CAD build for the part. Positions are in the model's coordinates, mm. Face numbers are marked on the shaded views. A direction names the side the tool comes from. Round coordinates to 2 decimals unless told otherwise and drop trailing zeros. Write each loop counter-clockwise with the first axis right and the second up, starting at its lowest first coordinate (ties: lowest second). Pieces come first, ordered by that corner, then holes. Notation, with made-up numbers: (-20.75, 75.25) - (22.25, 75.25) arc R20 ccw to (22.25, 109.25) - close; hole circle Ø1 at (30.5, 76). An arc over 180 degrees is marked (long way). Use one line per item in the form item = value. Start each with the question number.
Item 1: Pin check, flat tips, straight feed: pin 1 (1.8 mm diameter, centred on x = -13.5, z = 4, fed in from +Y); pin 2 (1.2 mm diameter, centred on x = -0.5, y = 1, fed in from -Z); pin 3 (0.8 mm diameter, centred on x = 1, y = 0.5, fed in from +Z). Stop position of each tip, or through.
Item 2: Band-saw the part on B-B, the plane z = 4. List the corners of the cut face in (x, y).
Item 3: Band-saw the part on D-D, the plane x = 6.5. List the corners of the cut face in (y, z).
Item 4: Band-saw the part on C-C, the plane x = 14.5. List the corners of the cut face in (y, z), and give its area (3 significant figures).
Item 5: Tool access for the marked faces 5, 6 and 7: list every direction of +Z, -Z, +X, -X, +Y, -Y with a clear straight run to the whole face (end or side of a thin tool).
Item 6: Band-saw the part on A-A, the plane x = -11.5. List the corners of the cut face in (y, z), and give its area (3 significant figures).
Item 7: Drill centre lines: L1, parallel to X at y = 7.5, z = 4.5; L2, parallel to Y at x = -4.3, z = 3; L3, parallel to Y at x = 6, z = 1.25. Where is each one in solid material? Low to high.
Item 8: Pull direction X, two halves, no side cores. Call the marked faces 1, 2, 3 and 4: +X half, -X half, draft (parallel to the pull), parting line (faces both ways), or undercut.
from build123d import *

# Parameters (mm, degrees)
EXTRUDE_1_DEPTH     = 6
CUT_EXTRUDE_1_DEPTH = 12.5
CUT_EXTRUDE_2_DEPTH = 12.5
SKETCH_4_R          = 1.5
CUT_EXTRUDE_3_DEPTH = 23.5
CUT_EXTRUDE_4_DEPTH = 2.5
FILLET_1_R          = 0.3


with BuildPart() as part:
    # 草图1 → 凸台-拉伸1 (new body)
    with BuildSketch(Plane.XY):
        Polygon((-17, 0), (17, 0), (17, 1.5), (5.5, 1.5), (5.5, 11.5), (4, 11.5), (4, 1.5), (-4, 1.5), (-4, 11.5), (-5.5, 11.5), (-5.5, 1.5), (-17, 1.5), align=None)
    extrude(amount=EXTRUDE_1_DEPTH)

    # 草图2 → 切除-拉伸1 (cut, through all)
    with BuildSketch(Plane.XZ):
        with BuildLine():
            Line((-14, 6), (-17, 6))
            Line((-17, 6), (-17, 3))
            ThreePointArc((-17, 3), (-16.121320344, 5.121320344), (-14, 6))
        make_face()
        with BuildLine():
            ThreePointArc((-14, 0), (-16.121320344, 0.878679656), (-17, 3))
            Line((-17, 3), (-17, 0))
            Line((-17, 0), (-14, 0))
        make_face()
        with BuildLine():
            Line((17, 0), (17, 3))
            ThreePointArc((17, 3), (16.121320344, 0.878679656), (14, 0))
            Line((14, 0), (17, 0))
        make_face()
        with BuildLine():
            Line((17, 6), (14, 6))
            ThreePointArc((14, 6), (16.121320344, 5.121320344), (17, 3))
            Line((17, 3), (17, 6))
        make_face()
    extrude(amount=-CUT_EXTRUDE_1_DEPTH, mode=Mode.SUBTRACT)

    # 草图3 → 切除-拉伸2 (cut, through all)
    with BuildSketch(Plane.XZ):
        with BuildLine():
            Line((-9, 1.5), (-14, 1.5))
            ThreePointArc((-14, 1.5), (-15.5, 3), (-14, 4.5))
            Line((-14, 4.5), (-9, 4.5))
            ThreePointArc((-9, 4.5), (-7.5, 3), (-9, 1.5))
        make_face()
        with BuildLine():
            Line((9, 4.5), (14, 4.5))
            ThreePointArc((14, 4.5), (15.5, 3), (14, 1.5))
            Line((14, 1.5), (9, 1.5))
            ThreePointArc((9, 1.5), (7.5, 3), (9, 4.5))
        make_face()
    extrude(amount=-CUT_EXTRUDE_2_DEPTH, mode=Mode.SUBTRACT)

    # 草图4 → 切除-拉伸3 (cut, through all)
    with BuildSketch(Plane(origin=(5.5, 0, 0), x_dir=(0, 0, -1), z_dir=(1, 0, 0))):
        with BuildLine():
            Line((-3, 11.5), (-6, 11.5))
            Line((-6, 11.5), (-6, 8.5))
            ThreePointArc((-6, 8.5), (-5.121320344, 10.621320344), (-3, 11.5))
        make_face()
        with BuildLine():
            Line((0, 11.5), (-3, 11.5))
            ThreePointArc((-3, 11.5), (-0.878679656, 10.621320344), (0, 8.5))
            Line((0, 8.5), (0, 11.5))
        make_face()
        with Locations((-3, 8.5)):
            Circle(SKETCH_4_R)
    extrude(amount=-CUT_EXTRUDE_3_DEPTH, mode=Mode.SUBTRACT)

    # 草图5 → 切除-拉伸4 (cut, through all)
    with BuildSketch(Plane(origin=(0, 1.5, 0), x_dir=(1, 0, 0), z_dir=(0, 1, 0))):
        Polygon((2.5, -1), (3.4, 0), (-3.4, 0), (-2.5, -1), align=None)
        Polygon((-3.4, -6), (3.4, -6), (2.5, -5), (-2.5, -5), align=None)
    extrude(amount=-CUT_EXTRUDE_4_DEPTH, mode=Mode.SUBTRACT)

    # 圆角1
    fillet_1_edges = [part.edges().sort_by_distance(p)[0] for p in [
        (-2.5, 0.75, 1),
        (-3.4, 0.75, 0),
        (3.4, 0.75, 0),
        (2.5, 0.75, 1),
        (-2.5, 0.75, 5),
        (2.5, 0.75, 5),
        (3.4, 0.75, 6),
        (-3.4, 0.75, 6),
    ]]
    fillet(fillet_1_edges, radius=FILLET_1_R)


solid = part.part
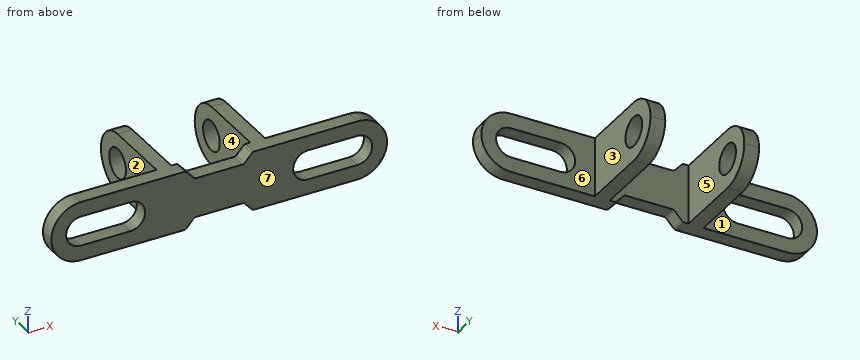
Determined:
q1.pin_1 = 1.5
q1.pin_2 = 1
q1.pin_3 = 5
q2.outline = (-16.83, 0) - (-15.12, 0) - (-15.12, 1.5) - (-16.83, 1.5) - close; (-7.88, 0) - (7.88, 0) - (7.88, 1.5) - (5.5, 1.5) - (5.5, 7.38) - (4, 7.38) - (4, 1.5) - (-4, 1.5) - (-4, 7.38) - (-5.5, 7.38) - (-5.5, 1.5) - (-7.88, 1.5) - close; (-5.5, 9.62) - (-4, 9.62) - (-4, 11.33) - (-5.5, 11.33) - close; (4, 9.62) - (5.5, 9.62) - (5.5, 11.33) - (4, 11.33) - close; (15.12, 0) - (16.83, 0) - (16.83, 1.5) - (15.12, 1.5) - close
q3.outline = (0, 0) - (1.5, 0) - (1.5, 6) - (0, 6) - close
q4.outline = (0, 0.04) - (1.5, 0.04) - (1.5, 1.59) - (0, 1.59) - close; (0, 4.41) - (1.5, 4.41) - (1.5, 5.96) - (0, 5.96) - close
q4.area = 4.63 mm²
q5.face_5 = +Z, -Z, +Y
q5.face_6 = +Z, -Z, +X, +Y
q5.face_7 = +Z, -Z, +X, -X, -Y
q6.outline = (0, 0) - (1.5, 0) - (1.5, 1.5) - (0, 1.5) - close; (0, 4.5) - (1.5, 4.5) - (1.5, 6) - (0, 6) - close
q6.area = 4.50 mm²
q7.L1 = -5.5 to -4, 4 to 5.5
q7.L2 = 0 to 7, 10 to 11.5
q7.L3 = 0 to 1.5
q8.face_1 = draft
q8.face_2 = -X half
q8.face_3 = +X half
q8.face_4 = undercut
